Build history of the part. All positions in model axes, mm. Face numbers are marked on the shaded views. A direction names the side the tool comes from. Coordinates: 2 decimals unless noted, no trailing zeros. Loops run counter-clockwise (first coordinate to the right, second up) from the corner with the lowest first, then second, coordinate; pieces in that order, holes last. Notation, with made-up numbers: (26.5, 1.5) - (74.5, 1.5) arc R26 ccw to (74.5, 17.5) - close; hole circle Ø4 at (80, 29). An arc over 180 degrees is marked (long way). One line per item, written item: value.
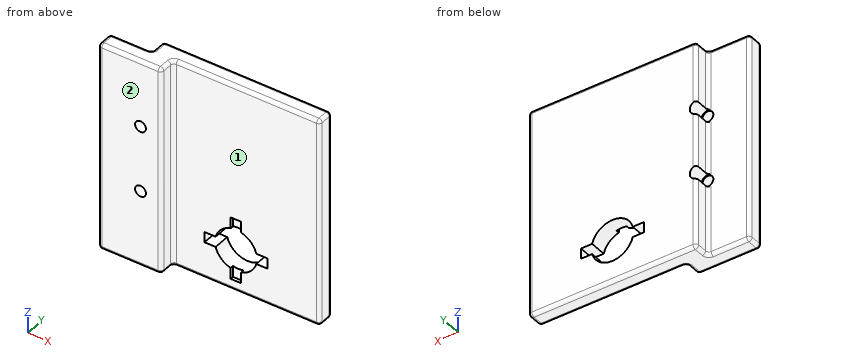
```python
from build123d import *

# Parameters (mm, degrees)
SKETCH1_W           = 63.5
SKETCH1_H           = 10
BOSS_EXTRUDE1_DEPTH = 63.5
SKETCH2_W           = 12.7
SKETCH2_H           = 63.5
CUT_EXTRUDE1_DEPTH  = 5
SKETCH3_W           = 44.45
SKETCH3_H           = 63.5
CUT_EXTRUDE2_DEPTH  = 5
SKETCH4_R           = 6.35
CUT_EXTRUDE3_DEPTH  = 5
SKETCH5_W           = 19.05
SKETCH5_H           = 3.175
CUT_EXTRUDE4_DEPTH  = 5
SKETCH6_R           = 2
CUT_EXTRUDE5_DEPTH  = 6
SKETCH7_R           = 1.65
CUT_EXTRUDE6_DEPTH  = 6
FILLET1_R           = 1
SKETCH8_W           = 3.18
SKETCH8_H           = 19.05
CUT_EXTRUDE7_DEPTH  = 1


with BuildPart() as part:
    # Sketch1 → Boss-Extrude1 (new body)
    with BuildSketch(Plane.XY):
        Rectangle(SKETCH1_W, SKETCH1_H)
    extrude(amount=BOSS_EXTRUDE1_DEPTH)

    # Sketch2 → Cut-Extrude1 (cut)
    with BuildSketch(Plane(origin=(0, 5, 0), x_dir=(1, 0, 0), z_dir=(0, 1, 0))):
        with Locations((-25.4, -31.75)):
            Rectangle(SKETCH2_W, SKETCH2_H)
    extrude(amount=-CUT_EXTRUDE1_DEPTH, mode=Mode.SUBTRACT)

    # Sketch3 → Cut-Extrude2 (cut)
    with BuildSketch(Plane.XZ.offset(5)):
        with Locations((9.525, 31.75)):
            Rectangle(SKETCH3_W, SKETCH3_H)
    extrude(amount=-CUT_EXTRUDE2_DEPTH, mode=Mode.SUBTRACT)

    # Sketch4 → Cut-Extrude3 (cut)
    with BuildSketch(Plane(origin=(0, 5, 0), x_dir=(1, 0, 0), z_dir=(0, 1, 0))):
        with Locations((6.35, -12.7)):
            Circle(SKETCH4_R)
    extrude(amount=-CUT_EXTRUDE3_DEPTH, mode=Mode.SUBTRACT)

    # Sketch5 → Cut-Extrude4 (cut)
    with BuildSketch(Plane.XZ):
        with Locations((6.35, 12.7)):
            Rectangle(SKETCH5_W, SKETCH5_H)
    extrude(amount=-CUT_EXTRUDE4_DEPTH, mode=Mode.SUBTRACT)

    # Sketch6 → Cut-Extrude5 (cut, through all)
    with BuildSketch(Plane(origin=(0, 0, 0), x_dir=(1, 0, 0), z_dir=(0, 1, 0))):
        with Locations((-19.05, -43.18)):
            Circle(SKETCH6_R)
        with Locations((-19.05, -23.18)):
            Circle(SKETCH6_R)
    extrude(amount=CUT_EXTRUDE5_DEPTH, mode=Mode.SUBTRACT)

    # Sketch7 → Cut-Extrude6 (cut, through all)
    with BuildSketch(Plane(origin=(0, 0, 0), x_dir=(1, 0, 0), z_dir=(0, 1, 0))):
        with Locations((-19.05, -23.18)):
            Circle(SKETCH7_R)
        with Locations((-19.05, -43.18)):
            Circle(SKETCH7_R)
    extrude(amount=-CUT_EXTRUDE6_DEPTH, mode=Mode.SUBTRACT)

    # Fillet1
    fillet1_edges = [part.edges().sort_by_distance(p)[0] for p in [
        (-31.75, -2.5, 0),
        (-22.225, -5, 63.5),
        (-31.75, -2.5, 63.5),
        (-19.05, 2.5, 0),
        (-19.05, 2.5, 63.5),
        (-19.05, 5, 54.34),
        (-31.75, 0, 31.75),
        (-25.4, 0, 0),
        (-19.05, 0, 10.59),
        (-25.4, 0, 63.5),
        (31.75, 2.5, 0),
        (31.75, 2.5, 63.5),
        (31.75, 0, 31.75),
        (9.525, 0, 0),
        (-12.7, 0, 31.75),
        (-12.7, -2.5, 0),
        (9.525, 0, 63.5),
        (-12.7, -2.5, 63.5),
        (-12.7, -5, 31.75),
        (-22.225, -5, 0),
        (6.35, 5, 0),
        (-31.75, -5, 31.75),
        (31.75, 5, 31.75),
        (6.35, 5, 63.5),
        (-19.05, 0, 33.18),
        (-19.05, 0, 54.34),
        (-19.05, 5, 33.18),
        (-19.05, 5, 10.59),
    ]]
    fillet(fillet1_edges, radius=FILLET1_R)

    # Sketch8 → Cut-Extrude7 (cut)
    with BuildSketch(Plane(origin=(0, 0, 0), x_dir=(-1, 0, 0), z_dir=(0, -1, 0))):
        with Locations((-6.35, -12.7)):
            Rectangle(SKETCH8_W, SKETCH8_H)
    extrude(amount=-CUT_EXTRUDE7_DEPTH, mode=Mode.SUBTRACT)


solid = part.part
```
Item 1: Cut at B-B, the plane x = -1. Write the cut outline in (y, z), then the cut area to 3 significant figures.
Check result:
outline: (0, 1) arc R1 ccw to (1, 0) - (4, 0) arc R1 ccw to (5, 1) - (5, 11.11) - (0, 11.11) - close; (0, 14.29) - (5, 14.29) - (5, 62.5) arc R1 ccw to (4, 63.5) - (1, 63.5) arc R1 ccw to (0, 62.5) - close
area: 301 mm^2
Item 2: Probe probe 1 along Z at (x, y) = (-19.05, -3.3); probe 2 along X at (y, z) = (-2.65, 43.18); probe 3 along Z at (x, y) = (-18, 4.25). List the from-to ranges inside material, lowest first. Write a range as from..to.
Check result:
probe 1: z = 0..21.53, 24.83..41.53, 44.83..63.5
probe 2: x = -31.75..-20.7, -17.4..-12.7
probe 3: z = 0.03..21.48, 24.88..41.48, 44.88..63.47
Item 3: Cut at A-A, the plane z = 23.18. Write the cut outline in (x, y), then the cut area to 3 significant figures.
Check result:
outline: (-31.75, -4) arc R1 ccw to (-30.75, -5) - (-20.7, -5) - (-20.7, 0) - (-30.75, 0) arc R1 ccw to (-31.75, -1) - close; (-17.4, -5) - (-13.7, -5) arc R1 ccw to (-12.7, -4) - (-12.7, -1) arc R1 cw to (-11.7, 0) - (30.75, 0) arc R1 ccw to (31.75, 1) - (31.75, 4) arc R1 ccw to (30.75, 5) - (-17.05, 5) - (-17.05, 0) - (-17.4, 0) - close
area: 322 mm^2
Item 4: Tool access for the marked faces 1 and 2: list every direction of +Z, -Z, +X, -X, +Y, -Y with a clear straight run to the whole face (end or side of a thin tool).
Check result:
face 1: +Z, -Z, +X, -Y
face 2: +Z, -Z, +X, -X, -Y
Item 5: Drop flat-ended pins along their axis: P1, Ø1, axis at y = -1.5, z = 13.5, coming from the +X side; P2, Ø6, axis at x = 6.5, z = 55.5, coming from the -Y side; P3, Ø3.5, axis at y = -2, z = 42.5, coming from the +X side. Give the stop position or say it passes through.
Check result:
P1: stops at x = -12.7
P2: stops at y = 0
P3: stops at x = -12.36
Item 6: Cut at D-D, the plane z = 49.5. Write the cut outline in (x, y).
Check result:
outline: (-31.75, -4) arc R1 ccw to (-30.75, -5) - (-13.7, -5) arc R1 ccw to (-12.7, -4) - (-12.7, -1) arc R1 cw to (-11.7, 0) - (30.75, 0) arc R1 ccw to (31.75, 1) - (31.75, 4) arc R1 ccw to (30.75, 5) - (-18.05, 5) arc R1 ccw to (-19.05, 4) - (-19.05, 1) arc R1 cw to (-20.05, 0) - (-30.75, 0) arc R1 ccw to (-31.75, -1) - close
